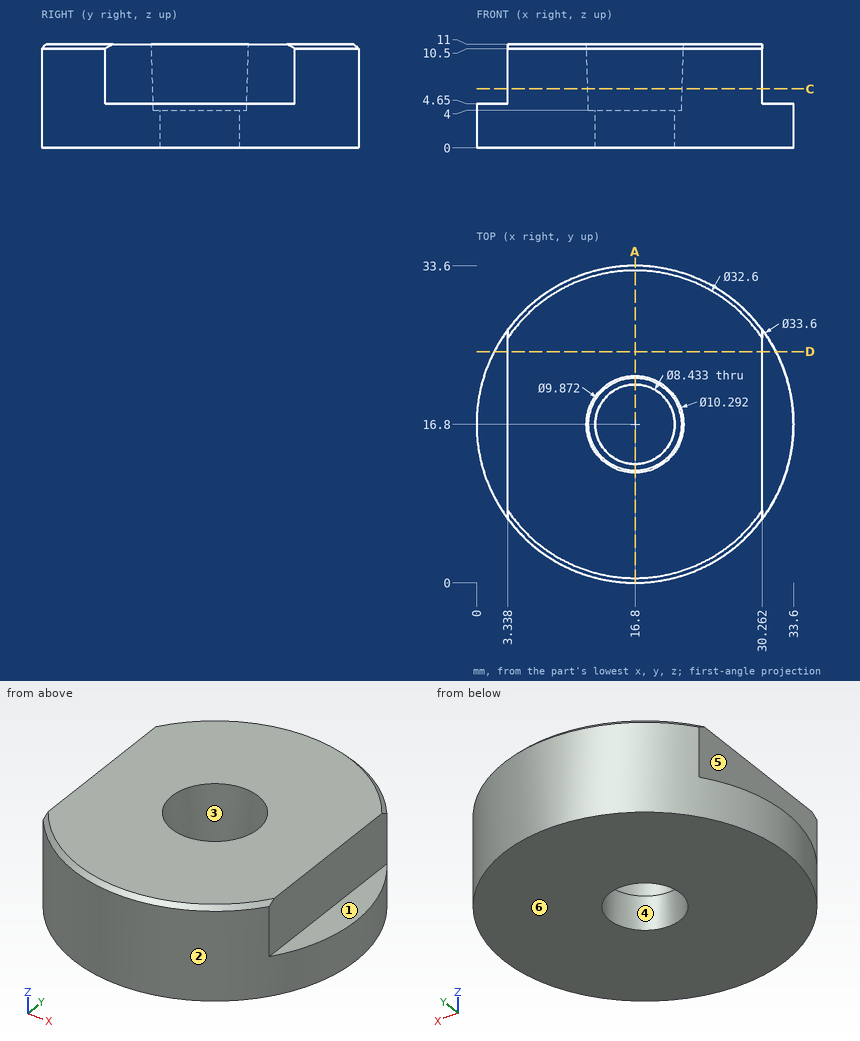
For this review, use the dimensioned drawing (mm, ordinates from the lowest corner) and the shaded views. A direction names the side the tool comes from. Give positions to 0.01 mm unless a question says otherwise; leave off trailing zeros. Write each loop counter-clockwise with the first axis right and the second up, starting at its lowest first coordinate (ties: lowest second). Pieces come first, ordered by that corner, then holes.
(1) Tool access review of the marked faces 1, 2 and 3: name each direction out of +Z, -Z, +X, -X, +Y, -Y from which nothing blocks a thin tool from reaching the whole face with its end or side.
(2) For P1, Ø9.5, axis at x = 16.8, y = 16.8, coming from the +Z side; P2, Ø3, axis at x = 18.5, z = 8.5, coming from the -Y side; P3, Ø4, axis at y = 10, z = 6.5, coming from the -X side (1 decimal), all flat-tipped, find the tip position at first contact; note any pin that passes through.
(3) Consider section C-C, the plane z = 6.25. Give the boundary of the cut face in (x, y), and give its area (3 significant figures).
(4) To check wall thickness, follow L1, parallel to X at y = 16.8, z = 2; L2, parallel to Y at x = 17, z = 4.5. State the ranges of each line that lie inside material, in increasing order.
(5) The part is to be moulded in two halves that separate along X. For the marked faces 4, 5 and 6, say which applies: released by +X, released by -X, zero draft, split by the parting line, or undercut.
(6) Consider section D-D, the plane y = 24.5. Give the boundary of the cut face in (x, z).
(7) Consider section A-A, the plane x = 16.8. Give the boundary of the cut face in (y, z) (1 decimal).
Returned:
1. face 1: +Z, +X, +Y, -Y
1. face 2: +Z, -Z
1. face 3: +Z
2. P1: stops at z = 4
2. P2: stops at y = 0
2. P3: stops at x = 1.1
3. outline: (3.34, 6.75) arc R16.8 ccw to (30.26, 6.75) - (30.26, 26.85) arc R16.8 ccw to (3.34, 26.85) - close; hole circle Ø10.01 at (16.8, 16.8)
3. area: 717 mm2
4. L1: x = 0 to 12.58, 21.02 to 33.6
4. L2: y = 0 to 11.85, 21.75 to 33.6
5. face 4: undercut
5. face 5: released by -X
5. face 6: zero draft
6. outline: (1.87, 0) - (31.73, 0) - (31.73, 4.65) - (30.26, 4.65) - (30.26, 11) - (3.34, 11) - (3.34, 4.65) - (1.87, 4.65) - close
7. outline: (0, 0) - (12.6, 0) - (12.6, 4) - (11.9, 4) - (11.7, 11) - (0.5, 11) - (0, 10.5) - close; (21, 0) - (33.6, 0) - (33.6, 10.5) - (33.1, 11) - (21.9, 11) - (21.7, 4) - (21, 4) - close
